Could you check a few things on this model? Use its own coordinates, in mm. A direction names the side the tool comes from. Coordinates: 2 decimals unless noted, no trailing zeros. Order: outer loops, then holes, each group sorted by start corner. A loop starts at its lowest first (then second) coordinate and runs counter-clockwise, first axis right, second up. Notation, with made-up numbers: (-10, 19) - (15, 19) arc R33 cw to (15, 51) - close; hole circle Ø6 at (-24, 65). An arc over 180 degrees is marked (long way). One line per item, written item: value.
from build123d import *

# Parameters (mm, degrees)
SKETCH2_W                    = 1.5875
SKETCH2_H                    = 82.55
BASE_FLANGE1_DEPTH           = 63.5
EDGE_FLANGE1_STRIP_W         = 7.8232
EDGE_FLANGE1_STRIP_H         = 1.5875
EDGE_FLANGE1_STRIP_CUT_DEPTH = 63.5
EDGE_FLANGE1_DEPTH           = 63.5
SKETCH10_R                   = 7
CUT_EXTRUDE1_DEPTH           = 105.73891424
EDGE_FLANGE2_STRIP_W         = 7.8232
EDGE_FLANGE2_STRIP_H         = 1.5875
EDGE_FLANGE2_STRIP_CUT_DEPTH = 63.5
EDGE_FLANGE2_DEPTH           = 63.5
EDGE_FLANGE3_STRIP_W         = 7.8232
EDGE_FLANGE3_STRIP_H         = 1.5875
EDGE_FLANGE3_STRIP_CUT_DEPTH = 63.5
EDGE_FLANGE3_DEPTH           = 63.5
EDGE_FLANGE4_STRIP_W         = 7.8232
EDGE_FLANGE4_STRIP_H         = 1.5875
EDGE_FLANGE4_STRIP_CUT_DEPTH = 63.5
EDGE_FLANGE4_DEPTH           = 63.5
SKETCH20_R                   = 7
CUT_EXTRUDE2_DEPTH           = 125.278268888


# Sheet-metal steps are written as plain solids
with BuildPart() as part:
    # Sketch2 → Base-Flange1 (new body)
    with BuildSketch(Plane.XY):
        with Locations((0.79375, 41.275)):
            Rectangle(SKETCH2_W, SKETCH2_H)
    extrude(amount=BASE_FLANGE1_DEPTH)

    # Edge-Flange1 strip (across the edge) → Edge-Flange1 strip cut (cut)
    with BuildSketch(Plane(origin=(0, 0, 0), x_dir=(0, 1, 0), z_dir=(0, 0, 1))):
        with Locations((-3.175, -0.79375)):
            Rectangle(EDGE_FLANGE1_STRIP_W, EDGE_FLANGE1_STRIP_H)
    extrude(amount=EDGE_FLANGE1_STRIP_CUT_DEPTH, mode=Mode.SUBTRACT)

    # Edge-Flange1 section (across the edge) → Edge-Flange1 (add)
    with BuildSketch(Plane(origin=(0, 0, 0), x_dir=(0, 1, 0), z_dir=(0, 0, 1))):
        with BuildLine():
            Line((-1.5875, 0.7366), (-1.5875, 11.1125))
            Line((-1.5875, 11.1125), (0, 11.1125))
            Line((0, 11.1125), (0, 0.7366))
            ThreePointArc((0, 0.7366), (0.215745145, 0.215745145), (0.7366, 0))
            Line((0.7366, 0), (0.7366, -1.5875))
            ThreePointArc((0.7366, -1.5875), (-0.90678687, -0.90678687), (-1.5875, 0.7366))
        make_face()
    extrude(amount=EDGE_FLANGE1_DEPTH)

    # Sketch10 → Cut-Extrude1 (cut, through all)
    with BuildSketch(Plane.ZY):
        with Locations((31.75, 63.4125)):
            Circle(SKETCH10_R)
    extrude(amount=-CUT_EXTRUDE1_DEPTH, mode=Mode.SUBTRACT)

    # Edge-Flange2 strip (across the edge) → Edge-Flange2 strip cut (cut)
    with BuildSketch(Plane(origin=(0, 82.55, 63.5), x_dir=(0, -1, 0), z_dir=(0, 0, -1))):
        with Locations((-3.175, -0.79375)):
            Rectangle(EDGE_FLANGE2_STRIP_W, EDGE_FLANGE2_STRIP_H)
    extrude(amount=EDGE_FLANGE2_STRIP_CUT_DEPTH, mode=Mode.SUBTRACT)

    # Edge-Flange2 section (across the edge) → Edge-Flange2 (add)
    with BuildSketch(Plane(origin=(0, 82.55, 63.5), x_dir=(0, -1, 0), z_dir=(0, 0, -1))):
        with BuildLine():
            Line((-1.5875, 0.7366), (-1.5875, 62.162499944))
            Line((-1.5875, 62.162499944), (0, 62.162499944))
            Line((0, 62.162499944), (0, 0.7366))
            ThreePointArc((0, 0.7366), (0.215745145, 0.215745145), (0.7366, 0))
            Line((0.7366, 0), (0.7366, -1.5875))
            ThreePointArc((0.7366, -1.5875), (-0.90678687, -0.90678687), (-1.5875, 0.7366))
        make_face()
    extrude(amount=EDGE_FLANGE2_DEPTH)

    # Edge-Flange3 strip (across the edge) → Edge-Flange3 strip cut (cut)
    with BuildSketch(Plane(origin=(-62.162499944, 82.55, 63.5), x_dir=(1, 0, 0), z_dir=(0, 0, -1))):
        with Locations((-3.175, -0.79375)):
            Rectangle(EDGE_FLANGE3_STRIP_W, EDGE_FLANGE3_STRIP_H)
    extrude(amount=EDGE_FLANGE3_STRIP_CUT_DEPTH, mode=Mode.SUBTRACT)

    # Edge-Flange3 section (across the edge) → Edge-Flange3 (add)
    with BuildSketch(Plane(origin=(-62.162499944, 82.55, 63.5), x_dir=(1, 0, 0), z_dir=(0, 0, -1))):
        with BuildLine():
            Line((-1.5875, 0.7366), (-1.5875, 82.55))
            Line((-1.5875, 82.55), (0, 82.55))
            Line((0, 82.55), (0, 0.7366))
            ThreePointArc((0, 0.7366), (0.215745145, 0.215745145), (0.7366, 0))
            Line((0.7366, 0), (0.7366, -1.5875))
            ThreePointArc((0.7366, -1.5875), (-0.90678687, -0.90678687), (-1.5875, 0.7366))
        make_face()
    extrude(amount=EDGE_FLANGE3_DEPTH)

    # Edge-Flange4 strip (across the edge) → Edge-Flange4 strip cut (cut)
    with BuildSketch(Plane(origin=(-62.162499944, 0, 63.5), x_dir=(0, 1, 0), z_dir=(0, 0, -1))):
        with Locations((-3.175, -0.79375)):
            Rectangle(EDGE_FLANGE4_STRIP_W, EDGE_FLANGE4_STRIP_H)
    extrude(amount=EDGE_FLANGE4_STRIP_CUT_DEPTH, mode=Mode.SUBTRACT)

    # Edge-Flange4 section (across the edge) → Edge-Flange4 (add)
    with BuildSketch(Plane(origin=(-62.162499944, 0, 63.5), x_dir=(0, 1, 0), z_dir=(0, 0, -1))):
        with BuildLine():
            Line((-1.5875, 0.7366), (-1.5875, 11.1125))
            Line((-1.5875, 11.1125), (0, 11.1125))
            Line((0, 11.1125), (0, 0.7366))
            ThreePointArc((0, 0.7366), (0.215745145, 0.215745145), (0.7366, 0))
            Line((0.7366, 0), (0.7366, -1.5875))
            ThreePointArc((0.7366, -1.5875), (-0.90678687, -0.90678687), (-1.5875, 0.7366))
        make_face()
    extrude(amount=EDGE_FLANGE4_DEPTH)

    # Sketch20 → Cut-Extrude2 (cut, through all)
    with BuildSketch(Plane(origin=(0, 84.1375, 0), x_dir=(1, 0, 0), z_dir=(0, 1, 0))):
        with Locations(Location((-32, -31.75, 0), (0, 0, 180))):
            Circle(SKETCH20_R)
    extrude(amount=-CUT_EXTRUDE2_DEPTH, mode=Mode.SUBTRACT)


solid = part.part
Item 1: If I drill on probe 1 along X at (y, z) = (38, 10); probe 2 along X at (y, z) = (82, 31); probe 3 along Y at (x, z) = (-55, 18.5), over which ranges is the centre line in solid material (lowest first)?
Conclusion:
probe 1: -63.75 to -62.16, 0 to 1.59
probe 2: -63.74 to -62.14, -0.02 to 1.58
probe 3: -1.59 to 0, 82.55 to 84.14
Item 2: I want a section at C-C on x = -32. Please give me the cut outline in (y, z).
Conclusion:
outline: (82.55, 0) - (84.14, 0) - (84.14, 24.75) - (82.55, 24.75) - close; (82.55, 38.75) - (84.14, 38.75) - (84.14, 63.5) - (82.55, 63.5) - close
Item 3: I'm going to push flat-ended pins straight in: pin 1 Ø8.5 at (x, z) = (-32, 31.75) entering from +Y; pin 2 Ø1 at (x, z) = (-49.5, 42) entering from -Y; pin 3 Ø1.3 at (y, z) = (-1, 28.5) entering from +X; pin 4 Ø1.3 at (y, z) = (-0.5, 27) entering from -X. Where does each tip first touch, or does it pass through?
Conclusion:
pin 1: through
pin 2: y = 82.55
pin 3: x = 1.32
pin 4: x = -63.67
Item 4: Thinking about a two-plate mould opening in Y: for faces 1 (the face through (0, 41, 31)), 2 (the face through (-63.75, 42, 32)), 3 (the face through (-62.162, 41, 32)), 4 (the face through (0.925, -0.889, 31.306)), which applies, pulls with the +Y half, pulls with the -Y half, needs draft (parallel to the pull), parting line crosses it, or undercut?
Conclusion:
face 1: undercut
face 2: needs draft
face 3: undercut
face 4: pulls with the -Y half
Item 5: I want a section at B-B on y = 24.5. Please give me the cut outline in (x, z).
Conclusion:
outline: (-63.75, 0) - (-62.16, 0) - (-62.16, 63.5) - (-63.75, 63.5) - close; (0, 0) - (1.59, 0) - (1.59, 63.5) - (0, 63.5) - close
Item 6: I want a section at A-A on z = 31.75. Please give me the cut outline in (x, y), then the cut area to 3 significant figures.
Conclusion:
outline: (-63.75, 0.74) arc R2.32 ccw to (-61.43, -1.59) - (-51.05, -1.59) - (-51.05, 0) - (-61.43, 0) arc R0.74 cw to (-62.16, 0.74) - (-62.16, 81.81) arc R0.74 cw to (-61.43, 82.55) - (-39, 82.55) - (-39, 84.14) - (-61.43, 84.14) arc R2.32 ccw to (-63.75, 81.81) - close; (-25, 82.55) - (-0.74, 82.55) arc R0.74 cw to (0, 81.81) - (0, 70.41) - (1.59, 70.41) - (1.59, 81.81) arc R2.32 ccw to (-0.74, 84.14) - (-25, 84.14) - close; (-11.11, -1.59) - (-0.74, -1.59) arc R2.32 ccw to (1.59, 0.74) - (1.59, 56.41) - (0, 56.41) - (0, 0.74) arc R0.74 cw to (-0.74, 0) - (-11.11, 0) - close
area: 358 mm²
Item 7: I want a section at D-D on z = 7. Please give me the cut outline in (x, y).
Conclusion:
outline: (-63.75, 0.74) arc R2.32 ccw to (-61.43, -1.59) - (-51.05, -1.59) - (-51.05, 0) - (-61.43, 0) arc R0.74 cw to (-62.16, 0.74) - (-62.16, 81.81) arc R0.74 cw to (-61.43, 82.55) - (-0.74, 82.55) arc R0.74 cw to (0, 81.81) - (0, 0.74) arc R0.74 cw to (-0.74, 0) - (-11.11, 0) - (-11.11, -1.59) - (-0.74, -1.59) arc R2.32 ccw to (1.59, 0.74) - (1.59, 81.81) arc R2.32 ccw to (-0.74, 84.14) - (-61.43, 84.14) arc R2.32 ccw to (-63.75, 81.81) - close
Item 8: For faces 5 (the face through (-24.8, 82.55, 32.2)), 6 (the face through (0.783, 57.202, 34.98)), 7 (the face through (-56, -1.588, 32)), which set-ups out of +Z, -Z, +X, -X, +Y, -Y let a thin tool reach every point of the face, with its end or its side?
Conclusion:
face 5: +Z, -Z
face 6: +X
face 7: +Z, -Z, +X, -X, -Y
